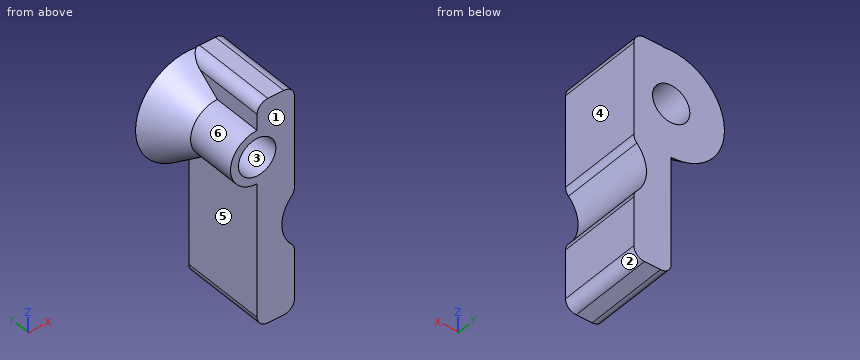
from build123d import *

# Parameters (mm, degrees)
F1_ANGLE_BACK = 90
F1_ANGLE      = 180
F4_DEPTH      = 8
F5_R          = 1.75
F6_DEPTH      = 25
F7_R          = 1
F8_R          = 1


with BuildPart() as f1:
    # F0 (on Top) → F1 (revolve)
    with BuildSketch(Plane.XY, mode=Mode.PRIVATE) as f1_sk:
        Polygon((0, 0), (0, 8), (-5, 8), (-1, 2.6666666667), (-1, 0), align=None)
    revolve(f1_sk.sketch.rotate(Axis((0, 4, 0), (0, 1, 0)), -F1_ANGLE_BACK), axis=Axis((0, 4, 0), (0, 1, 0)), revolution_arc=F1_ANGLE)

    # F3 (on Front) → F4 (join)
    with BuildSketch(Plane.XZ):
        with BuildLine():
            Line((3.5, 5.0001256168), (0, 5.0001256168))
            Line((0, 5.0001256168), (0, 2.5))
            ThreePointArc((0, 2.5), (-2.5, 0), (0, -2.5))
            Line((0, -2.5), (0, -15.9998743832))
            Line((0, -15.9998743832), (3.5, -15.9998743832))
            Line((3.5, -15.9998743832), (3.5, -9.9998743832))
            ThreePointArc((3.5, -9.9998743832), (2.3136093185, -7.4998743832), (3.5, -4.9998743832))
            Line((3.5, -4.9998743832), (3.5, 5.0001256168))
        make_face()
    extrude(amount=-F4_DEPTH)

    # F5 (on face) → F6 (cut)
    with BuildSketch(Plane(origin=(0, 8, 0), x_dir=(-1, 0, 0), z_dir=(0, 1, 0))):
        Circle(F5_R)
    extrude(amount=-F6_DEPTH, mode=Mode.SUBTRACT)

    # F7
    f7_edges = [f1.edges().sort_by_distance(p)[0] for p in [
        (3.5, 4, 5.000126),
        (0, 4, -15.999874),
        (3.5, 4, -15.999874),
        (3.5, 4, -9.999874),
        (3.5, 4, -4.999874),
    ]]
    fillet(f7_edges, radius=F7_R)

    # F8
    f8_edges = [f1.edges().sort_by_distance(p)[0] for p in [
        (0, 4, 5.000126),
    ]]
    fillet(f8_edges, radius=F8_R)


solid = f1.part
Can you work these out from the model? Positions are in its coordinate system, mm. Face numbers are marked on the shaded views. A direction names the side the tool comes from. Round coordinates to 2 decimals unless told otherwise and drop trailing zeros. Write each loop counter-clockwise with the first axis right and the second up, starting at its lowest first coordinate (ties: lowest second). Pieces come first, ordered by that corner, then holes. Notation, with made-up numbers: (-30.75, 62.25) -> (8.25, 62.25) arc R9 cw to (8.25, 67.25) -> close; hole circle Ø6 at (3, 5). An arc over 180 degrees is marked (long way). Use one line per item in the form item = value. Start each with the question number.
Q1. Imagine slicing it at C-C (y = 5). Please give me the cut outline in (x, z), then the cut area to 3 significant figures.
Q2. Imagine slicing it at B-B (y = 3.5). Please give me the cut outline in (x, z), then the cut area to 3 significant figures.
Q3. I'm going to push flat-ended pins straight in: P1, Ø0.5, axis at y = 2, z = 3, coming from the -X side; P2, Ø2, axis at x = -3, y = 4.5, coming from the -Z side. Where does each tip first touch, or does it pass through?
Q4. We'd pull the mould along X, two halves only. Please class the marked faces 1, 2 and 3: +X half, -X half, draft (parallel to the pull), parting line (faces both ways), or undercut.
Q5. Imagine slicing it at D-D (z = -9.5). Please give me the cut outline in (x, y).
Q6. Which directions (+Z, -Z, +X, -X, +Y, -Y) give clear straight access to the entire face, cutting with the end or side of a thin tool? Please do the marked faces 4, 5 and 6.
Q7. If I drill on probe 1 along X at (y, z) = (4.25, -3); probe 2 along Z at (x, y) = (2.75, 2.5); probe 3 along Z at (x, y) = (-1.25, 6), over which ranges is the centre line in solid material (lowest first)? Write a range as [from, to].
Q8. Imagine slicing it at A-A (z = 0). Please give me the cut outline in (x, y), then the cut area to 3 significant figures.
Worked out:
q1.outline = (0, -15) arc R1 ccw to (1, -16) -> (2.5, -16) arc R1 ccw to (3.5, -15) -> (3.5, -10.44) arc R1 ccw to (3.22, -9.74) arc R3.23 cw to (3.22, -5.26) arc R1 ccw to (3.5, -4.56) -> (3.5, 4) arc R1 ccw to (2.5, 5) -> (1, 5) arc R1 ccw to (0, 4) -> (0, 2.75) arc R2.75 ccw to (0, -2.75) -> close; hole circle Ø3.5 at (0, 0)
q1.area = 70.7 mm^2
q2.outline = (0, -15) arc R1 ccw to (1, -16) -> (2.5, -16) arc R1 ccw to (3.5, -15) -> (3.5, -10.44) arc R1 ccw to (3.22, -9.74) arc R3.23 cw to (3.22, -5.26) arc R1 ccw to (3.5, -4.56) -> (3.5, 4) arc R1 ccw to (2.5, 5) -> (1, 5) arc R1 ccw to (0, 4) -> (0, 2.5) arc R2.5 ccw to (0, -2.5) -> close; hole circle Ø3.5 at (0, 0)
q2.area = 68.7 mm^2
q3.P1 = 0
q3.P2 = -1.78
q4.face_1 = draft
q4.face_2 = +X half
q4.face_3 = undercut
q5.outline = (0, 0) -> (3.01, 0) -> (3.01, 8) -> (0, 8) -> close
q6.face_4 = +Z, -Z, +X, +Y, -Y
q6.face_5 = -Z, -X, -Y
q6.face_6 = -X, -Y
q7.probe_1 = [0, 3.5]
q7.probe_2 = [-15.97, -9.12], [-5.88, 4.97]
q7.probe_3 = [-3.27, -1.22], [1.22, 3.27]
q8.outline = (-5, 8) -> (-2.5, 4.67) -> (-2.5, 0) -> (-1.75, 0) -> (-1.75, 8) -> close; (1.75, 0) -> (3.5, 0) -> (3.5, 8) -> (1.75, 8) -> close
q8.area = 24.2 mm^2
